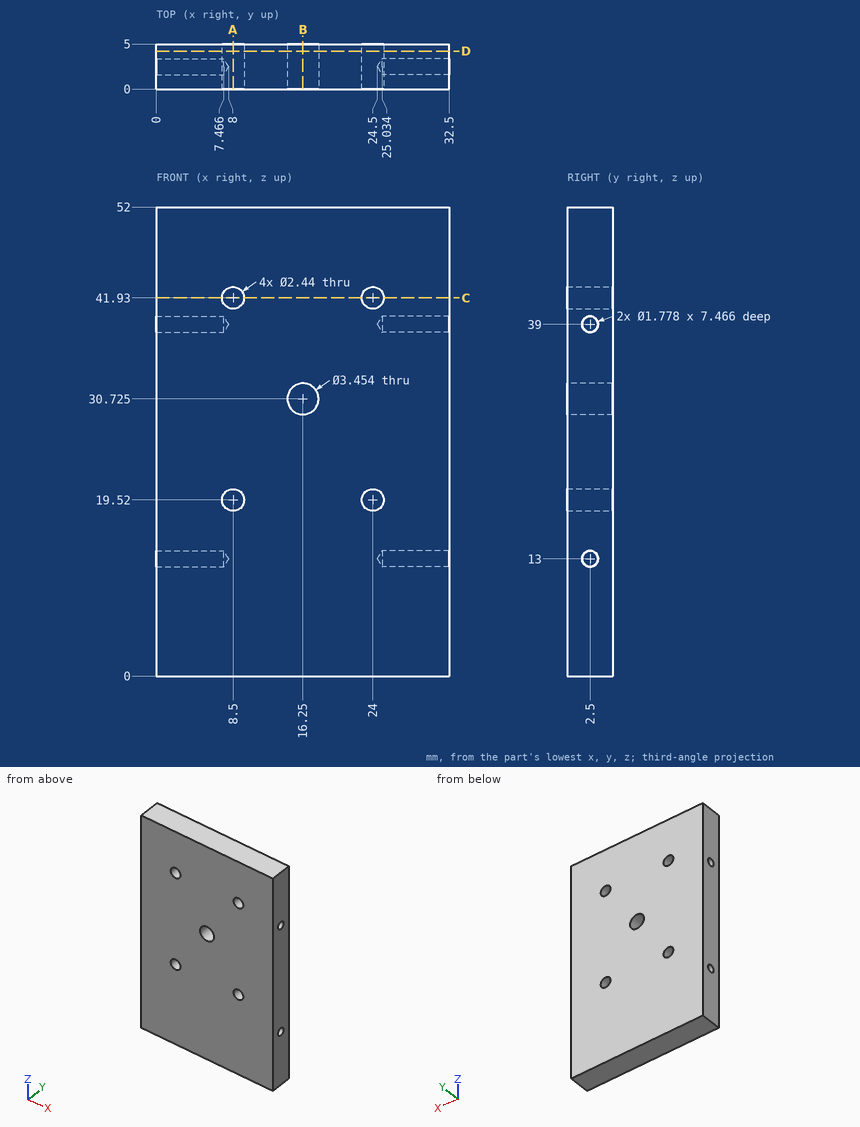
Answer from the drawing. Dimensions are ordinates in mm from the lowest x, y and z of the part. Round coordinates to 2 decimals unless told otherwise and drop trailing zeros. Write each loop counter-clockwise with the first axis right and the second up, starting at its lowest first coordinate (ties: lowest second). Pieces come first, ordered by that corner, then holes.
1. Straight lines are drawn through the part: L1, parallel to Z at x = 2, y = 2.5; L2, parallel to Z at x = 8.5, y = 3.65; L3, parallel to Y at x = 30, z = 13. For each, find the intervals that lie inside material, in ascending order.
2. The part is cut by section B-B, the plane x = 16.25. Determine the outline of the cut face in (y, z).
3. Given pin 1 Ø1.4 at (y, z) = (2.5, 13) entering from +X; pin 2 Ø2 at (x, z) = (24, 41.93) entering from -Y; pin 3 Ø1.6 at (y, z) = (2.5, 13) entering from -X, each flat-ended and moving along its own axis, determine where each tip first touches the part or whether it passes through.
4. The part is cut by section A-A, the plane x = 8.5. Determine the outline of the cut face in (y, z).
5. The part is cut by section C-C, the plane z = 41.93. Determine the outline of the cut face in (x, y), then the cut area to 3 significant figures.
6. The part is cut by section D-D, the plane y = 4.2. State how many separate pieces and enclosed holes the cut face has, then the cut area to 3 significant figures.
Values:
1. L1: z = 0 to 12.11, 13.89 to 38.11, 39.89 to 52
1. L2: z = 0 to 18.3, 20.74 to 40.71, 43.15 to 52
1. L3: y = 0 to 1.61, 3.39 to 5
2. outline: (0, 0) - (5, 0) - (5, 29) - (0, 29) - close; (0, 32.45) - (5, 32.45) - (5, 52) - (0, 52) - close
3. pin 1: stops at x = 24.92
3. pin 2: passes through
3. pin 3: stops at x = 7.52
4. outline: (0, 0) - (5, 0) - (5, 18.3) - (0, 18.3) - close; (0, 20.74) - (5, 20.74) - (5, 40.71) - (0, 40.71) - close; (0, 43.15) - (5, 43.15) - (5, 52) - (0, 52) - close
5. outline: (0, 0) - (7.28, 0) - (7.28, 5) - (0, 5) - close; (9.72, 0) - (22.78, 0) - (22.78, 5) - (9.72, 5) - close; (25.22, 0) - (32.5, 0) - (32.5, 5) - (25.22, 5) - close
5. area: 138 mm2
6. separate pieces: 1
6. enclosed holes: 5
6. area: 1,660 mm2
